Geometry check sheet. Reference: the model listing, model coordinates, mm. Face numbers are marked on the shaded views. A direction names the side the tool comes from. Coordinates: 2 decimals unless noted, no trailing zeros. Loops run counter-clockwise (first coordinate to the right, second up) from the corner with the lowest first, then second, coordinate; pieces in that order, holes last. Notation, with made-up numbers: (31, 67) - (38, 67) arc R11 cw to (38, 80) - close; hole circle Ø9 at (-7, 39). An arc over 180 degrees is marked (long way). Write each question's results on one line, items separated by ' | '. Start each with the question number.
(1) Sectioned sample at B-B (z = 8). Enter the section's corners in (x, y), plus the area to 3 significant figures.
(2) Mould release check, pull along Y, two halves, no side actions. Record for the marked faces 1, 2 and 3: pulls with the +Y half, pulls with the -Y half, needs draft (parallel to the pull), parting line crosses it, or undercut.
(3) Go/stop test with flat-tipped pins: pin 1 Ø12 at (y, z) = (-4.5, 15.5) entering from -X; pin 2 Ø1.5 at (x, y) = (17.5, 7) entering from +Z; pin 3 Ø1 at (y, z) = (-9.5, 2) entering from -X; pin 4 Ø4 at (x, z) = (-19, 5) entering from -Y. Record where each tip stops, or that it passes through.
(4) Sectioned sample at C-C (z = 2). Enter the section's corners in (x, y), plus the area to 3 significant figures.
(5) Sectioned sample at D-D (y = 25). Enter the section's corners in (x, z), plus the area to 3 significant figures.
(6) Material ranges on probe 1 along X at (y, z) = (-3, 19); probe 2 along X at (y, z) = (-9.5, 16); probe 3 along X at (y, z) = (-4.5, 8.25), recorded low to high.
(7) Sectioned sample at A-A (x = 0). Enter the section's corners in (y, z), plus the area to 3 significant figures.
(8) Access from +Z, -Z, +X, -X, +Y, -Y to the whole of each face (thin tool, end or side, straight path). Record for the marked faces 4 and 5.
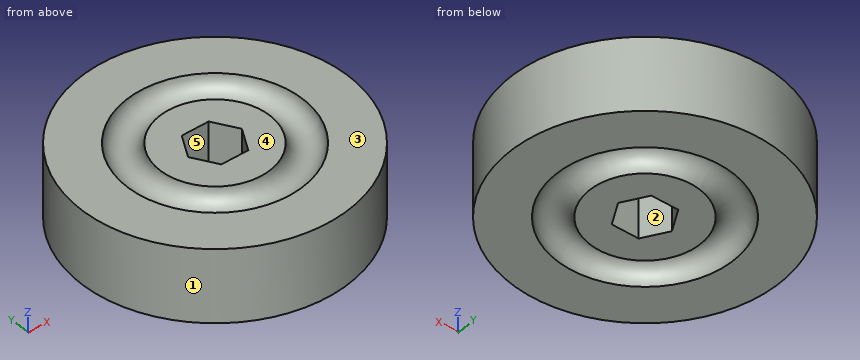
from build123d import *

# Parameters (mm, degrees)
SKETCH1_R           = 36.5
BOSS_EXTRUDE1_DEPTH = 20


with BuildPart() as part:
    # Sketch1 → Boss-Extrude1 (new body)
    with BuildSketch(Plane.XY):
        Circle(SKETCH1_R)
        Polygon((7.493, 0), (3.7465, 6.489128351), (-3.7465, 6.489128351), (-7.493, 0), (-3.7465, -6.489128351), (3.7465, -6.489128351), align=None, mode=Mode.SUBTRACT)
    extrude(amount=BOSS_EXTRUDE1_DEPTH)

    # Cut-Sweep2: sweep along a path in Sketch3
    with BuildLine(Plane(origin=(0, 0, 0), x_dir=(-1, 0, 0), z_dir=(0, 0, -1))) as cut_sweep2_path:
        CenterArc((0, 0), 19.5, 0, 360)
    # Sketch2 → Cut-Sweep2 (sweep, cut)
    with BuildSketch(Plane(origin=(0, 0, 0), x_dir=(1, 0, 0), z_dir=(0, 1, 0))):
        with BuildLine():
            Line((-24, 0), (-15, 0))
            ThreePointArc((-15, 0), (-19.5, -4.5), (-24, 0))
        make_face()
    cut_sweep2 = sweep(path=cut_sweep2_path.line, mode=Mode.SUBTRACT)

    # Mirror1: Cut-Sweep2 across plane
    add(cut_sweep2.mirror(Plane.XY.offset(10)), mode=Mode.SUBTRACT)


solid = part.part
Outcome:
1) outline: circle Ø73 at (0, 0); hole (-7.49, 0) - (-3.75, -6.49) - (3.75, -6.49) - (7.49, 0) - (3.75, 6.49) - (-3.75, 6.49) - close | area: 4,040 mm2
2) face 1: parting line crosses it | face 2: undercut | face 3: needs draft
3) pin 1: stops at x = -36.5 | pin 2: stops at z = 15.72 | pin 3: stops at x = -35.37 | pin 4: stops at y = -32.3
4) outline: circle Ø73 at (0, 0); circle Ø30.94 at (0, 0); hole circle Ø47.06 at (0, 0); hole (-7.49, 0) - (-3.75, -6.49) - (3.75, -6.49) - (7.49, 0) - (3.75, 6.49) - (-3.75, 6.49) - close | area: 3,050 mm2
5) outline: (-26.59, 0) - (26.59, 0) - (26.59, 20) - (-26.59, 20) - close | area: 1,060 mm2
6) probe 1: x = -36.38 to -23.7, -14.81 to -5.76, 5.76 to 14.81, 23.7 to 36.38 | probe 2: x = -35.24 to -19.36, -14.62 to 14.62, 19.36 to 35.24 | probe 3: x = -36.22 to -4.89, 4.89 to 36.22
7) outline: (-36.5, 0) - (-24, 0) arc R4.5 cw to (-15, 0) - (-6.49, 0) - (-6.49, 20) - (-15, 20) arc R4.5 cw to (-24, 20) - (-36.5, 20) - close; (6.49, 0) - (15, 0) arc R4.5 cw to (24, 0) - (36.5, 0) - (36.5, 20) - (24, 20) arc R4.5 cw to (15, 20) - (6.49, 20) - close | area: 1,070 mm2
8) face 4: +Z, +X, -X, +Y, -Y | face 5: +Z, -Z
